Geometry check sheet. Reference: the model listing, model coordinates, mm. A direction names the side the tool comes from. Round coordinates to 2 decimals unless told otherwise and drop trailing zeros. Loops run counter-clockwise (first coordinate to the right, second up) from the corner with the lowest first, then second, coordinate; pieces in that order, holes last. Notation, with made-up numbers: (70.5, 88.5) - (111.5, 88.5) arc R29 cw to (111.5, 112.5) - close; hole circle Ø7 at (81, -33). An arc over 180 degrees is marked (long way). Write item = value, one per line.
```python
from build123d import *

# Parameters (mm, degrees)
F0_W     = 127
F0_H     = 111.125
F1_DEPTH = 88.9
F2_W     = 34.925
F2_H     = 34.925
F3_DEPTH = 31.75
F4_W     = 44.45
F4_H     = 44.45
F5_DEPTH = 25.4
F7_DEPTH = 6.35
F8_W     = 12.7
F8_H     = 12.7
F9_DEPTH = 41.275
F10_R    = 0.8255


with BuildPart() as f1:
    # F0 (on Top) → F1 (new body)
    with BuildSketch(Plane.XY):
        Rectangle(F0_W, F0_H)
    extrude(amount=F1_DEPTH)

    # F2 (on face) → F3 (join)
    with BuildSketch(Plane.XY.offset(88.9)):
        with Locations((46.0375, -38.1)):
            Rectangle(F2_W, F2_H)
    extrude(amount=F3_DEPTH)

    # F4 (on face) → F5 (join)
    with BuildSketch(Plane.XY.offset(120.65)):
        with Locations((46.0375, -38.1)):
            Rectangle(F4_W, F4_H)
    extrude(amount=F5_DEPTH)

    # F6 (on face) → F7 (join)
    with BuildSketch(Plane.XY.offset(146.05)):
        Polygon((60.0175166498, -52.0800166498), (65.8082291484, -38.1), (60.0175166498, -24.1199833502), (46.0375, -18.3292708516), (32.0574833502, -24.1199833502), (26.2667708516, -38.1), (32.0574833502, -52.0800166498), (46.0375, -57.8707291484), align=None)
    extrude(amount=F7_DEPTH)

    # F8 (on face) → F9 (join)
    with BuildSketch(Plane.XY.offset(88.9)):
        with Locations((-51.5943879418, 26.04008)):
            Rectangle(F8_W, F8_H)
        with Locations((-13.4957394752, 26.04008)):
            Rectangle(F8_W, F8_H)
    extrude(amount=F9_DEPTH)

    # F10
    f10_edges = [f1.edges().sort_by_distance(p)[0] for p in [
        (-17.4625, -55.5625, 88.9),
        (-63.5, 0, 88.9),
        (-63.5, -55.5625, 44.45),
        (28.575, -55.5625, 104.775),
        (63.5, -55.5625, 60.325),
        (28.575, -20.6375, 104.775),
        (23.8125, -15.875, 133.35),
        (23.8125, -60.325, 133.35),
        (68.2625, -60.325, 133.35),
        (46.0375, -60.325, 120.65),
        (23.8125, -38.1, 120.65),
        (46.0375, -60.325, 146.05),
        (23.8125, -38.1, 146.05),
        (68.2625, -38.1, 146.05),
        (46.0375, -15.875, 146.05),
        (53.027508, -21.224627, 152.4),
        (62.912873, -31.109992, 152.4),
        (62.912873, -45.090008, 152.4),
        (53.027508, -54.975373, 152.4),
        (39.047492, -54.975373, 152.4),
        (29.162127, -45.090008, 152.4),
        (29.162127, -31.109992, 152.4),
        (39.047492, -21.224627, 152.4),
        (32.057483, -52.080017, 149.225),
        (46.0375, -57.870729, 149.225),
        (26.266771, -38.1, 149.225),
        (60.017517, -52.080017, 149.225),
        (65.808229, -38.1, 149.225),
        (60.017517, -24.119983, 149.225),
        (46.0375, -18.329271, 149.225),
        (32.057483, -24.119983, 149.225),
        (68.2625, -15.875, 133.35),
        (63.5, -20.6375, 104.775),
        (68.2625, -38.1, 120.65),
        (46.0375, -15.875, 120.65),
        (63.5, 17.4625, 88.9),
        (0, 55.5625, 88.9),
        (63.5, 55.5625, 44.45),
        (-57.944388, 32.39008, 109.5375),
        (-45.244388, 32.39008, 109.5375),
        (-57.944388, 19.69008, 109.5375),
        (-57.944388, 26.04008, 130.175),
        (-51.594388, 32.39008, 130.175),
        (-45.244388, 26.04008, 130.175),
        (-51.594388, 19.69008, 130.175),
        (-19.845739, 32.39008, 109.5375),
        (-7.145739, 32.39008, 109.5375),
        (-19.845739, 26.04008, 130.175),
        (-13.495739, 32.39008, 130.175),
        (-7.145739, 26.04008, 130.175),
        (-13.495739, 19.69008, 130.175),
        (-19.845739, 19.69008, 109.5375),
        (-7.145739, 19.69008, 109.5375),
        (-45.244388, 19.69008, 109.5375),
        (-63.5, 55.5625, 44.45),
        (63.5, 0, 0),
        (0, 55.5625, 0),
        (0, -55.5625, 0),
        (-63.5, 0, 0),
    ]]
    fillet(f10_edges, radius=F10_R)


solid = f1.part
```
(1) Gauge pin test, flat ends, axial feed: pin 1 (7 mm diameter, centred on y = -41, z = 128.5, fed in from -X); pin 2 (6 mm diameter, centred on x = -12, y = -40.5, fed in from +Z); pin 3 (12 mm diameter, centred on y = 23.5, z = 118, fed in from +X). Record the tip position at first contact, or that the pin passes through.
Answers follow:
pin_1 = 23.81
pin_2 = 88.9
pin_3 = -7.15
(2) Section check A-A (x = -25.5). Enter the section's corners in (y, z), then the cut area to 3 significant figures.
Answers follow:
outline = (-55.56, 0.83) arc R0.83 ccw to (-54.74, 0) - (54.74, 0) arc R0.83 ccw to (55.56, 0.83) - (55.56, 88.07) arc R0.83 ccw to (54.74, 88.9) - (-54.74, 88.9) arc R0.83 ccw to (-55.56, 88.07) - close
area = 9,880 mm²
(3) Section check C-C (z = 56). Enter the section's corners in (x, y).
Answers follow:
outline = (-63.5, -54.74) arc R0.83 ccw to (-62.67, -55.56) - (62.67, -55.56) arc R0.83 ccw to (63.5, -54.74) - (63.5, 54.74) arc R0.83 ccw to (62.67, 55.56) - (-62.67, 55.56) arc R0.83 ccw to (-63.5, 54.74) - close
(4) Set-up check for faces 1 (the flat face through (-57.944, 26, 109)), 2 (the flat face through (46, -15.875, 133)), 3 (the flat face through (38.954, -54.937, 148.774)): record each of +Z, -Z, +X, -X, +Y, -Y from which the full face is reachable in a straight line by a thin tool's end or side.
Answers follow:
face_1 = +Z, -X, +Y, -Y
face_2 = +Z, +X, -X, +Y
face_3 = +Z, -X, -Y
(5) Scan lines: L1, parallel to X at y = 43, z = 75; L2, parallel to Y at x = 4.5, z = 81; L3, parallel to Z at x = -56, y = 17. Record each from-to range of solid material in increasing order. Write a range as [from, to].
Answers follow:
L1 = [-63.5, 63.5]
L2 = [-55.56, 55.56]
L3 = [0, 88.9]
(6) Section check B-B (y = 22.5). Enter the section's corners in (x, z) (1 decimal), then the cut area to 3 significant figures.
Answers follow:
outline = (-63.5, 0.8) arc R0.8 ccw to (-62.7, 0) - (62.7, 0) arc R0.8 ccw to (63.5, 0.8) - (63.5, 88.1) arc R0.8 ccw to (62.7, 88.9) - (-7.1, 88.9) - (-7.1, 129.3) arc R0.8 ccw to (-8, 130.2) - (-19, 130.2) arc R0.8 ccw to (-19.8, 129.3) - (-19.8, 88.9) - (-45.2, 88.9) - (-45.2, 129.3) arc R0.8 ccw to (-46.1, 130.2) - (-57.1, 130.2) arc R0.8 ccw to (-57.9, 129.3) - (-57.9, 88.9) - (-62.7, 88.9) arc R0.8 ccw to (-63.5, 88.1) - close
area = 12,300 mm²
(7) Section check D-D (x = -51). Enter the section's corners in (y, z) (1 decimal), then the cut area to 3 significant figures.
Answers follow:
outline = (-55.6, 0.8) arc R0.8 ccw to (-54.7, 0) - (54.7, 0) arc R0.8 ccw to (55.6, 0.8) - (55.6, 88.1) arc R0.8 ccw to (54.7, 88.9) - (32.4, 88.9) - (32.4, 129.3) arc R0.8 ccw to (31.6, 130.2) - (20.5, 130.2) arc R0.8 ccw to (19.7, 129.3) - (19.7, 88.9) - (-54.7, 88.9) arc R0.8 ccw to (-55.6, 88.1) - close
area = 10,400 mm²
(8) Mould release check, pull along Z, two halves, no side actions. Record for faces 4 (the cylindrical face through (39.04, -21.48, 152.15)), 5 (the flat face through (27, -38, 120.65)), 6 (the flat face through (-45.244, 26, 109)): pulls with the +Z half, pulls with the -Z half, needs draft (parallel to the pull), parting line crosses it, or undercut.
Answers follow:
face_4 = pulls with the +Z half
face_5 = undercut
face_6 = needs draft
